Geometry check sheet. Reference: the model listing, model coordinates, mm. Face numbers are marked on the shaded views. A direction names the side the tool comes from. Give positions to 0.01 mm unless a question says otherwise; leave off trailing zeros. Loops run counter-clockwise (first coordinate to the right, second up) from the corner with the lowest first, then second, coordinate; pieces in that order, holes last. Notation, with made-up numbers: (-25.75, 19) -> (17.25, 19) arc R21 cw to (17.25, 48) -> close; hole circle Ø9 at (34.25, 69.5). An arc over 180 degrees is marked (long way). Answer as a JSON object with one key per item and string values.
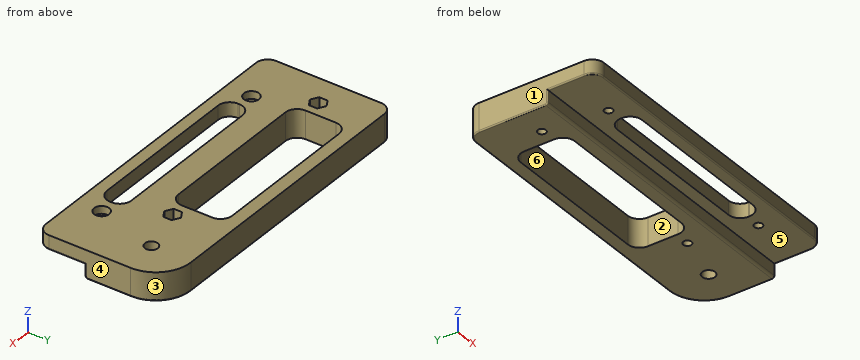
Autodesk Fusion 360 part; units mm, degrees
sketch "Sketch1" plane through (0, 0, 0) normal (0, 0, 1) x (1, 0, 0)
  line L0 (67.5, 27.5) -> (-67.5, 27.5)
  line L1 (-67.5, 27.5) -> (-67.5, -27.5)
  line L2 (-67.5, -27.5) -> (67.5, -27.5)
  line L3 (67.5, -27.5) -> (67.5, 27.5)
  line L4 (67.5, 27.5) -> (-67.5, -27.5) construction
  line L5 (-67.5, 27.5) -> (67.5, -27.5) construction
  dimension "d1" = 55
  dimension "d2" = 135
extrude "Extrude1" add sketch "Sketch1" along normal blind 6
sketch "Sketch3" plane through (0, 0, 0) normal (0, 0, -1) x (-1, 0, 0)
  line L0 (-67.5, 27.5) -> (-67.5, -27.5)
  line L1 (-67.5, -27.5) -> (67.5, -27.5)
  line L2 (67.5, -27.5) -> (67.5, 27.5)
  line L3 (67.5, 27.5) -> (-67.5, 27.5)
  line L4 (-67.5, -7) -> (67.5, -7)
  line L5 (67.5, -7) -> (67.5, 27.5)
  line L6 (67.5, 27.5) -> (-67.5, 27.5)
  line L7 (-67.5, 27.5) -> (-67.5, -7)
  line L8 (-67.5, -7) -> (67.5, 27.5) construction
  line L9 (67.5, -7) -> (-67.5, 27.5) construction
  point P0 (0, 10.25)
  dimension "d14" = 34.5
  dimension "d30" = 20.5
extrude "Extrude2" add sketch "Sketch3" along normal blind 6 contours L0 L2 L3 L4 L5 L6 L7
sketch "Sketch2" plane through (0, 0, 6) normal (0, 0, 1) x (1, 0, 0)
  line L0 (67.5, -27.5) -> (67.5, 27.5)
  line L1 (67.5, 27.5) -> (-67.5, 27.5)
  line L2 (-67.5, 27.5) -> (-67.5, -27.5)
  line L3 (-67.5, -27.5) -> (67.5, -27.5)
  line L4 (67.5, -7) -> (-67.5, -7)
  point P0 (-44.5, -16.5)
  point P1 (44.5, -16.5)
  dimension "d7" = 23
  dimension "d47" = 9.5
  dimension "d48" = 9.5
  dimension "d49" = 89
hole "Hole1" at (-44.5, -16.5, 6) at (44.5, -16.5, 6) direction (0, 0, -1) diameter 3.5 end through all counterbore diameter 6.5 counterbore depth 3.25
sketch "Sketch4" plane through (0, 0, -6) normal (0, 0, -1) x (-1, 0, 0)
  line L0 (-67.5, 27.5) -> (-67.5, -7)
  line L1 (-67.5, -7) -> (67.5, -7)
  line L2 (67.5, -7) -> (67.5, 27.5)
  line L3 (67.5, 27.5) -> (-67.5, 27.5)
  line L4 (-67.5, 4.75) -> (67.5, 4.75) construction
  point P0 (54.75, 4.75)
  point P1 (-31.75, 4.75)
  dimension "d19" = 12.75
  dimension "d20" = 86.5
  dimension "d31" = 11.75
hole "Hole2" at (31.75, 4.75, -6) at (-54.75, 4.75, -6) direction (0, 0, 1) diameter 3.5 end through all
sketch "Sketch5" plane through (0, 0, 6) normal (0, 0, 1) x (1, 0, 0)
  circle A0 centre (31.75, 4.75) radius 1.75
  circle A1 centre (-54.75, 4.75) radius 1.75
  circle A2 centre (-44.5, -16.5) radius 3.25
  circle A3 centre (44.5, -16.5) radius 3.25
  line L0 (67.5, -27.5) -> (67.5, 27.5)
  line L1 (67.5, 27.5) -> (-67.5, 27.5)
  line L2 (-67.5, 27.5) -> (-67.5, -27.5)
  line L3 (-67.5, -27.5) -> (67.5, -27.5)
  line L4 (-51.65, 6.5398) -> (-54.75, 8.3296)
  line L5 (-54.75, 8.3296) -> (-57.85, 6.5398)
  line L6 (-57.85, 6.5398) -> (-57.85, 2.9602)
  line L7 (-57.85, 2.9602) -> (-54.75, 1.1704)
  line L8 (-54.75, 1.1704) -> (-51.65, 2.9602)
  line L9 (-51.65, 2.9602) -> (-51.65, 6.5398)
  line L10 (34.85, 2.9602) -> (34.85, 6.5398)
  line L11 (34.85, 6.5398) -> (31.75, 8.3296)
  line L12 (31.75, 8.3296) -> (28.65, 6.5398)
  line L13 (28.65, 6.5398) -> (28.65, 2.9602)
  line L14 (28.65, 2.9602) -> (31.75, 1.1704)
  line L15 (31.75, 1.1704) -> (34.85, 2.9602)
  point P0 (-54.75, 4.75)
  point P1 (31.75, 4.75)
  dimension "d24" = 6.2
  dimension "d25" = 6.2
extrude "Extrude3" cut sketch "Sketch5" against normal blind 6 contours L4 L5 L6 L7 L8 L9 | L10 L11 L12 L13 L14 L15
sketch "Sketch6" plane through (0, 0, -6) normal (0, 0, -1) x (-1, 0, 0)
  circle A0 centre (-31.75, 4.75) radius 1.75
  circle A1 centre (54.75, 4.75) radius 1.75
  line L0 (-67.5, 27.5) -> (-67.5, -7)
  line L1 (-67.5, -7) -> (67.5, -7)
  line L2 (67.5, -7) -> (67.5, 27.5)
  line L3 (67.5, 27.5) -> (-67.5, 27.5)
  line L4 (59.5, -7) -> (-36.5, -7) construction
  line L5 (-36.5, -7) -> (-36.5, 28) construction
  line L6 (-36.5, 28) -> (59.5, 28) construction
  line L7 (59.5, 28) -> (59.5, -7) construction
  line L8 (59.5, -7) -> (-36.5, 28) construction
  line L9 (-36.5, -7) -> (59.5, 28) construction
  line L10 (11.5, 50.5144) -> (11.5, -41.0982) construction
  line L11 (-52, 27.5) -> (-52, -7) construction
  line L12 (-36.5, 10.25) -> (-67.5, 10.25) construction
  point P0 (11.5, 10.5)
  point P1 (-52, 10.25)
  dimension "d28" = 35
  dimension "d29" = 96
hole "Hole3" at (52, 10.25, -6) direction (0, 0, 1) diameter 5.5 end through all
fillet "Fillet1" radius 5 2 edges at (67.5, -27.5, 3) (-67.5, -27.5, 3)
fillet "Fillet1" radius 5 1 edges at (-67.5, 27.5, 0)
fillet "Fillet3" radius 15 1 edges at (67.5, 27.5, 0)
fillet "Fillet4" radius 1 1 edges at (0, -7, -6)
fillet "Fillet5" radius 0.5 14 edges at (-67.5, -14.75, 0) (-66.0355, -26.0355, 0) (0, -27.5, 0) (66.0355, -26.0355, 0) (67.5, -14.75, 0) (-67.5, -7, -2.5) (-67.5, -6.7071, -5.7071) (-67.5, 8.25, -6) (-66.0355, 26.0355, -6) (-5, 27.5, -6) (63.1066, 23.1066, -6) (67.5, 3.25, -6) (67.5, -6.7071, -5.7071) (67.5, -7, -2.5)
sketch "Sketch7" plane through (0, 0, -6) normal (0, 0, -1) x (-1, 0, 0)
  line L0 (-67, 12.5) -> (-67, -6)
  line L1 (-67, -6) -> (67, -6)
  line L2 (67, -6) -> (67, 22.5)
  arc A0 (67, 22.5) -> (62.5, 27) centre (62.5, 22.5) ccw
  line L3 (62.5, 27) -> (-52.5, 27)
  arc A1 (-52.5, 27) -> (-67, 12.5) centre (-52.5, 12.5) ccw
  circle A2 centre (54.75, 4.75) radius 1.75
  circle A3 centre (-31.75, 4.75) radius 1.75
  circle A4 centre (-52, 10.25) radius 2.75
  line L4 (-25.25, 22) -> (48.25, 22)
  line L5 (48.25, 22) -> (48.25, -1)
  line L6 (48.25, -1) -> (-25.25, -1)
  line L7 (-25.25, -1) -> (-25.25, 22)
  line L8 (-25.25, 22) -> (48.25, -1) construction
  line L9 (48.25, 22) -> (-25.25, -1) construction
  point P0 (11.5, 10.5)
  dimension "d50" = 5
  dimension "d51" = 5
  dimension "d52" = 6.5
  dimension "d53" = 6.5
extrude "Extrude4" cut sketch "Sketch7" against normal through all contours L4 L5 L6 L7
fillet "Fillet6" radius 5 4 edges at (25.25, 22, 0) (25.25, -1, 0) (-48.25, -1, 0) (-48.25, 22, 0)
sketch "Sketch8" plane through (0, 0, 0) normal (0, 0, -1) x (-1, 0, 0)
  line L0 (-67, -7) -> (-67, -22.5)
  arc A0 (-67, -22.5) -> (-62.5, -27) centre (-62.5, -22.5) ccw
  line L1 (-62.5, -27) -> (62.5, -27)
  arc A1 (62.5, -27) -> (67, -22.5) centre (62.5, -22.5) ccw
  line L2 (67, -22.5) -> (67, -7)
  line L3 (67, -7) -> (-67, -7)
  circle A2 centre (-44.5, -16.5) radius 1.75
  circle A3 centre (44.5, -16.5) radius 1.75
  line L4 (38, -22.5) -> (-38, -22.5)
  line L5 (-38, -22.5) -> (-38, -12)
  line L6 (-38, -12) -> (38, -12)
  line L7 (38, -12) -> (38, -22.5)
  line L8 (38, -22.5) -> (-38, -12) construction
  line L9 (-38, -22.5) -> (38, -12) construction
  line L10 (-62.5, -27.5) -> (62.5, -27.5)
  point P0 (0, -17.25)
  dimension "d57" = 5
  dimension "d58" = 5
  dimension "d59" = 6.5
  dimension "d60" = 6.5
extrude "Extrude5" cut sketch "Sketch8" against normal through all contours L4 L5 L6 L7
fillet "Fillet7" radius 5 4 edges at (38, -12, 3) (38, -22.5, 3) (-38, -22.5, 3) (-38, -12, 3)
equation "d7 = 21.5 mm + 1.5 mm"
equation "d19 = 15 mm - 2.25 mm"
equation "d20 = 82 mm + 4.5 mm"
equation "d25 = d24"
equation "d31 = 9.5 mm + 2.25 mm"
equation "d51 = d50"
equation "d53 = d52"
equation "d58 = d57"
equation "d60 = d59"
1) Section check B-B on x = -8. Record the cut outline in (y, z).
Geometry check:
{"outline": "(-27.5, 0.5) arc R0.5 ccw to (-27, 0) -> (-22.5, 0) -> (-22.5, 6) -> (-27.5, 6) -> close; (-12, 0) -> (-7, 0) -> (-7, -5) arc R1 ccw to (-6, -6) -> (-1, -6) -> (-1, 6) -> (-12, 6) -> close; (22, -6) -> (27, -6) arc R0.5 ccw to (27.5, -5.5) -> (27.5, 6) -> (22, 6) -> close"}
2) Section check A-A on y = 10.25. Record the cut outline in (x, z).
Geometry check:
{"outline": "(-67.5, -5.5) arc R0.5 ccw to (-67, -6) -> (-48.25, -6) -> (-48.25, 6) -> (-67.5, 6) -> close; (25.25, -6) -> (49.25, -6) -> (49.25, 6) -> (25.25, 6) -> close; (54.75, -6) -> (67, -6) arc R0.5 ccw to (67.5, -5.5) -> (67.5, 6) -> (54.75, 6) -> close"}
3) Tool access check on the marked faces 4, 5 and 6. Record the directions out of +Z, -Z, +X, -X, +Y, -Y that give a thin tool (end or side, any length) a straight path to the whole face; none if there is none.
Geometry check:
{"face 4": "+Z, -Z, +X, +Y, -Y", "face 5": "-Z, +X, -X, -Y", "face 6": "+Z, -Z"}
4) Depth check by flat-ended pin: P1, Ø10, axis at x = 13.5, y = -19.5, coming from the -Z side; P2, Ø2.5, axis at x = 22, z = -2, coming from the -Y side. Enter the tip coordinate at first touch or a pass-through.
Geometry check:
{"P1": "stops at z = 0", "P2": "stops at y = -7"}
5) Material ranges on line 1 along Y through (x, z) = (-4, 3.25); line 2 along X through (y, z) = (-16.5, 1.4); line 3 along X through (y, z) = (10.25, -0.25), recorded low to high. Write a range as from..to.
Geometry check:
{"line 1": "y = -27.5..-22.5, -12..-1, 22..27.5", "line 2": "x = -67.5..-46.25, -42.75..-37.97, 37.97..42.75, 46.25..67.5", "line 3": "x = -67.5..-48.25, 25.25..49.25, 54.75..67.5"}
6) Section check C-C on x = 44.5. Record the cut outline in (y, z), plus the area to 3 significant figures.
Geometry check:
{"outline": "(-27.5, 0.5) arc R0.5 ccw to (-27, 0) -> (-18.25, 0) -> (-18.25, 2.75) -> (-19.75, 2.75) -> (-19.75, 6) -> (-27.5, 6) -> close; (-14.75, 0) -> (-7, 0) -> (-7, -5) arc R1 ccw to (-6, -6) -> (27, -6) arc R0.5 ccw to (27.5, -5.5) -> (27.5, 6) -> (-13.25, 6) -> (-13.25, 2.75) -> (-14.75, 2.75) -> close", "area": "506 mm2"}
7) Draft check along Y on the marked faces 1, 2 and 3. Enter one of: pulls with the +Y half, pulls with the -Y half, needs draft (parallel to the pull), parting line crosses it, or undercut.
Geometry check:
{"face 1": "needs draft", "face 2": "undercut", "face 3": "pulls with the +Y half"}
